Geometry: final body of the model. Coordinates: model frame, mm. Face numbers are marked on the shaded views. A direction names the side the tool comes from. Give positions to 0.01 mm unless a question says otherwise; leave off trailing zeros. Write each loop counter-clockwise with the first axis right and the second up, starting at its lowest first coordinate (ties: lowest second). Pieces come first, ordered by that corner, then holes. Notation, with made-up numbers: M -35,60.25 L -8,60.25 A18 cw -8,71.25 Z; hole C 4,13 d4. An arc over 180 degrees is marked long. One line per question, with ' | ' between items.
from build123d import *

# Parameters (mm, degrees)
SKETCH_1_R           = 7.5
EXTRUDE_1_DEPTH      = 15
EXTRUDE_2_DEPTH      = 10
EXTRUDE_2_DEPTH_BACK = 10
EXTRUDE_3_DEPTH      = 35
EXTRUDE_3_DEPTH_BACK = 35
SKETCH_3_R           = 5


with BuildPart() as part:
    # Эскиз1 → Бобышка-Вытянуть1 (new body)
    with BuildSketch(Plane.XY):
        Circle(SKETCH_1_R)
    extrude(amount=EXTRUDE_1_DEPTH)

    # Эскиз2 → Бобышка-Вытянуть2 (add, two sides: drawn at the far end of the back side and taken through both)
    with BuildSketch(Plane(origin=(0, 0, 0), x_dir=(0, 0, -1), z_dir=(1, 0, 0)).offset(-EXTRUDE_2_DEPTH_BACK)):
        with BuildLine():
            Line((-15, 10), (-25, 10))
            ThreePointArc((-25, 10), (-35, 0), (-25, -10))
            Line((-25, -10), (-15, -10))
            Line((-15, -10), (-15, 10))
        make_face()
    extrude(amount=EXTRUDE_2_DEPTH + EXTRUDE_2_DEPTH_BACK)

    # Эскиз3 → Бобышка-Вытянуть3 (add, two sides: drawn at the far end of the back side and taken through both)
    with BuildSketch(Plane(origin=(0, 0, 0), x_dir=(0, 0, -1), z_dir=(1, 0, 0)).offset(-EXTRUDE_3_DEPTH_BACK)):
        with Locations((-25, 0)):
            Circle(SKETCH_3_R)
    extrude(amount=EXTRUDE_3_DEPTH + EXTRUDE_3_DEPTH_BACK)


solid = part.part
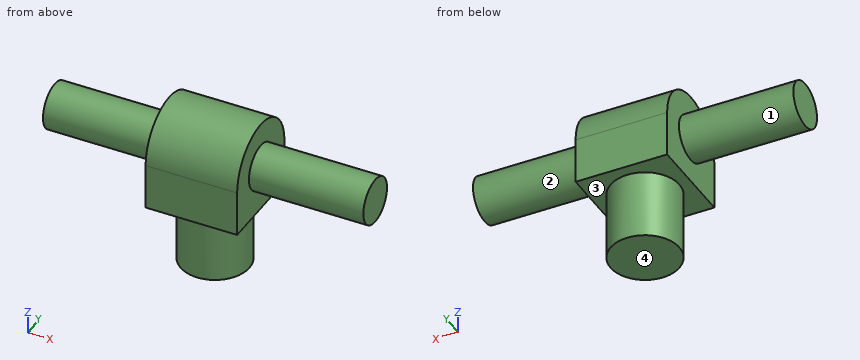
(1) Cut plane D-D, the plane y = -3.5. Return loops of the section in (x, z), then the cut area to 3 significant figures.
Working result:
outline: M -35,21.43 L -10,21.43 L -10,15 L -6.63,15 L -6.63,0 L 6.63,0 L 6.63,15 L 10,15 L 10,21.43 L 35,21.43 L 35,28.57 L 10,28.57 L 10,34.37 L -10,34.37 L -10,28.57 L -35,28.57 Z | area: 943 mm^2
(2) First-contact query: P1, Ø4, axis at x = -19, z = 20, coming from the +Y side; P2, Ø2, axis at y = -4, z = 20, coming from the +X side; P3, Ø2, axis at x = 6.5, y = -5, coming from the +Z side. Flat tips, straight axial feed; report the tip coordinate or a pass-through.
Working result:
P1: stops at y = 4 | P2: stops at x = 10 | P3: stops at z = 34.17
(3) Cut plane C-C, the plane z = 26. Return loops of the section in (x, y).
Working result:
outline: M -35,-4.9 L -10,-4.9 L -10,-9.95 L 10,-9.95 L 10,-4.9 L 35,-4.9 L 35,4.9 L 10,4.9 L 10,9.95 L -10,9.95 L -10,4.9 L -35,4.9 Z
(4) Cut plane A-A, the plane y = 0. Return loops of the section in (x, z), then the cut area to 4 significant figures.
Working result:
outline: M -35,20 L -10,20 L -10,15 L -7.5,15 L -7.5,0 L 7.5,0 L 7.5,15 L 10,15 L 10,20 L 35,20 L 35,30 L 10,30 L 10,35 L -10,35 L -10,30 L -35,30 Z | area: 1,125 mm^2
(5) Cut plane B-B, the plane x = 0. Return loops of the section in (y, z).
Working result:
outline: M -10,15 L -7.5,15 L -7.5,0 L 7.5,0 L 7.5,15 L 10,15 L 10,25 A10 ccw -10,25 Z
(6) Set-up query: the marked faces 1, 2, 3 and 4. Return all of +Z, -Z, +X, -X, +Y, -Y with unobstructed straight access to the full face (end or side cutting, diameter ignored); none if empty.
Working result:
face 1: -X | face 2: +X | face 3: -Z | face 4: -Z, +X, -X, +Y, -Y
(7) Material intervals for L1, parallel to X at y = 3, z = 18.5; L2, parallel to Z at x = 27.5, y = -0.25; L3, parallel to Z at x = 28, y = 1, sorted ascending. Write a range as [from, to].
Working result:
L1: x = [-10, 10] | L2: z = [20.01, 29.99] | L3: z = [20.1, 29.9]
